from build123d import *

# Parameters (mm, degrees)
BOSS_EXTRUDE1_DEPTH = 6.35


with BuildPart() as part:
    # Sketch1 → Boss-Extrude1 (new body)
    with BuildSketch(Plane(origin=(0, 0, 0), x_dir=(1, 0, 0), z_dir=(0, 1, 0))):
        with BuildLine():
            Line((9.525, -3.175), (-9.525, -3.175))
            Line((-9.525, -3.175), (-9.525, 3.175))
            Line((-9.525, 3.175), (-19.05, 3.175))
            Line((-19.05, 3.175), (-19.05, 28.575))
            ThreePointArc((-19.05, 28.575), (-15.330256121, 37.555256121), (-6.35, 41.275))
            Line((-6.35, 41.275), (6.35, 41.275))
            ThreePointArc((6.35, 41.275), (15.330256121, 37.555256121), (19.05, 28.575))
            Line((19.05, 28.575), (19.05, 3.175))
            Line((19.05, 3.175), (9.525, 3.175))
            Line((9.525, 3.175), (9.525, -3.175))
        make_face()
    extrude(amount=BOSS_EXTRUDE1_DEPTH)


solid = part.part
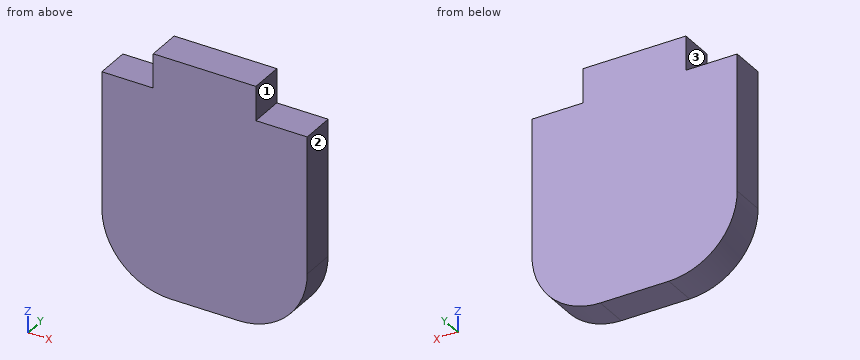
Input: part model. Units: mm. Frame: model coordinates. Face numbers are marked on the shaded views. A direction names the side the tool comes from. Round coordinates to 2 decimals unless told otherwise and drop trailing zeros. Order: outer loops, then holes, each group sorted by start corner. A loop starts at its lowest first (then second) coordinate and runs counter-clockwise, first axis right, second up. Notation, with made-up numbers: (7.5, 18) - (16.5, 18) arc R28 ccw to (16.5, 36) - close; hole circle Ø6 at (9, 12.25). An arc over 180 degrees is marked (long way). Answer as a JSON object with one key per item and string values. Group by question number.
(1) Cut plane C-C (z = -38). Return loops of the section in (x, y), then the cut area to 3 significant figures.
(2) Material intervals for probe 1 along X at (y, z) = (5.25, 1) (3 decimals); probe 2 along Z at (x, y) = (-17, 4.75) (3 decimals); probe 3 along Z at (x, y) = (8, 4.75) (3 decimals), sorted ascending. Write a range as from..to.
(3) Pin query (flat end, axial travel): P1, Ø1.5, axis at x = 10, y = 1.5, coming from the -Z side; P2, Ø3, axis at x = -12.5, y = 3, coming from the +Z side (3 decimals). Return the tip coordinate at first contact, or that it passes through.
(4) Cut plane B-B (x = 14). Return loops of the section in (y, z) (3 decimals), then the cut area to 3 significant figures.
(5) Cut plane A-A (y = 3.75). Return loops of the section in (x, z) (3 decimals).
(6) Reachability of the marked faces 1, 2 and 3 from +Z, -Z, +X, -X, +Y, -Y: full face, straight path, thin tool, end or side. Return the list, or none.
Here are the results:
{
 "1": {"outline": "(-14.86, 0) - (14.86, 0) - (14.86, 6.35) - (-14.86, 6.35) - close", "area": "189 mm^2"},
 "2": {"probe 1": "x = -9.525..9.525", "probe 2": "z = -35.494..-3.175", "probe 3": "z = -41.167..3.175"},
 "3": {"P1": "stops at z = -40.94", "P2": "stops at z = -3.175"},
 "4": {"outline": "(0, -38.712) - (6.35, -38.712) - (6.35, -3.175) - (0, -3.175) - close", "area": "226 mm^2"},
 "5": {"outline": "(-19.05, -28.575) arc R12.7 ccw to (-6.35, -41.275) - (6.35, -41.275) arc R12.7 ccw to (19.05, -28.575) - (19.05, -3.175) - (9.525, -3.175) - (9.525, 3.175) - (-9.525, 3.175) - (-9.525, -3.175) - (-19.05, -3.175) - close"},
 "6": {"face 1": "+Z, +X, +Y, -Y", "face 2": "+Z, -Z, +X, +Y, -Y", "face 3": "+Z, -X, +Y, -Y"}
}
